Source: CAD feature listing. Evaluate the final solid. Frame: model axes, mm. A direction names the side the tool comes from. Give positions to 0.01 mm unless a question says otherwise; leave off trailing zeros. Write each loop counter-clockwise with the first axis right and the second up, starting at its lowest first coordinate (ties: lowest second). Pieces come first, ordered by that corner, then holes. Notation, with made-up numbers: (50.25, 32.5) -> (61.25, 32.5) arc R18 cw to (61.25, 37.5) -> close; hole circle Ø11 at (37.25, -36). An arc over 180 degrees is marked (long way). Use a Markdown table: item, result. Add a question column.
Autodesk Inventor part; units mm, degrees
ref_plane "Work Plane1" through (0, -12.5, 0) normal (0, -1, 0) x (1, 0, 0)
ref_plane "YZ Plane" through (0, 0, 0) normal (1, 0, 0) x (0, 1, 0)
ref_plane "XZ Plane" through (0, 0, 0) normal (0, 1, 0) x (-1, 0, 0)
sketch "Sketch1" plane through (0, 0, 0) normal (0, 1, 0) x (-1, 0, 0)
  line L0 (0, 0) -> (-150, 0)
  line L1 (-150, 0) -> (-150, -20) construction
  line L2 (-150, -20) -> (0, -37.6327)
  line L3 (0, -37.6327) -> (0, 0) construction
  arc A0 (-150, 0) -> (-150, -20) centre (-150, -10) ccw
  arc A1 (0, -37.6327) -> (0, 0) centre (-6.7783, -18.8163) ccw
  dimension "d0" = 150
  dimension "d1" = 20
  dimension "d3" = 20
extrude "Extrusion1" add sketch "Sketch1" along normal blind 5
sketch "Sketch5" plane through (0, 5, 0) normal (0, 1, 0) x (1, 0, 0)
  line L0 (0, 7) -> (40.3, 7)
  line L1 (40.3, 7) -> (40.3, 27)
  line L2 (40.3, 27) -> (0, 27)
  line L3 (0, 27) -> (0, 7)
  line L4 (0, 0) -> (150, 0)
  arc A0 (0, 37.6327) -> (0, 0) centre (6.7783, 18.8163) ccw
  line L5 (0, 0) -> (0, 37.6327) construction
  dimension "d13" = 40.3
  dimension "d14" = 20
  dimension "d15" = 7
  dimension "d16" = 0
extrude "Extrusion3" cut sketch "Sketch5" against normal blind 5
ref_plane "Work Plane1" through (0, -12.5, 0) normal (0, -1, 0) x (1, 0, 0)
mirror "Mirror1" about plane through (0, -12.5, 0) normal (0, -1, 0) of "Extrusion1"
sketch "Sketch8" plane through (0, 0, 0) normal (0, 0, 1) x (1, 0, 0)
  line L0 (0, 0) -> (40.3, 0)
  line L1 (0, -25) -> (150, -25)
  line L2 (0, 0) -> (40.3767, 0)
  line L3 (40.3767, 0) -> (40.3767, -25)
  line L4 (40.3767, -25) -> (0, -25)
  line L5 (0, -25) -> (0, 0)
extrude "Extrusion4" add sketch "Sketch8" against normal blind 5
sketch "Sketch11" plane through (0, 5, 0) normal (0, 1, 0) x (1, 0, 0)
  circle A0 centre (-3.8458, 11.9975) radius 2
  circle A1 centre (-3.8458, 11.9975) radius 2
  circle A2 centre (-3.8458, 21.9992) radius 2
  circle A3 centre (44.2605, 21.9992) radius 2
  circle A4 centre (-3.8458, 21.9992) radius 2
  circle A5 centre (44.2605, 11.9975) radius 2
  circle A6 centre (44.2605, 21.9992) radius 2
  circle A7 centre (44.2605, 11.9975) radius 2
  point P0 (0, 0)
extrude "Extrusion6" cut sketch "Sketch11" against normal blind 5
sketch "Sketch14" plane through (0, 0, -37.6327) normal (0.1167, 0, -0.9932) x (-0.9932, 0, -0.1167)
  line L0 (-151.0328, -25) -> (0, -25)
  line L1 (-4.3935, 0) -> (-44.3935, 0)
  line L2 (-44.3935, 0) -> (-44.3935, -25)
  line L3 (-44.3935, -25) -> (-4.3935, -25)
  line L4 (-4.3935, -25) -> (-4.3935, 0)
  dimension "d31" = 40
extrude "Extrusion7" add sketch "Sketch14" against normal blind 5
sketch "Sketch17" plane through (0, 5, 0) normal (0, 1, 0) x (1, 0, 0)
  arc A0 (150, 0) -> (150, 20) centre (150, 10) ccw
  line L0 (150, 20) -> (44.0899, 32.4499)
  line L1 (150, 0) -> (150, 20)
  point P0 (0, 0)
extrude "Extrusion10" add sketch "Sketch17" against normal up to surface (35 mm away)
sketch "Sketch18" plane through (0, -30, 0) normal (0, -1, 0) x (1, 0, 0)
  circle A0 centre (10.7396, -16.9983) radius 5
  circle A1 centre (10.7396, -16.9983) radius 2.9
  point P0 (0, 0)
  dimension "d42" = 10
extrude "Extrusion11" add sketch "Sketch18" along normal blind 6 contours A0 | A1
properties part number "Tibia" material "PVC, Unplasticized"
(1) Cut plane A-A on y = -3. Return the cut outline in (x, z), then the cut area to 3 significant figures.
(2) Cut plane B-B on x = 72. Return the cut outline in (y, z).
(3) Material intervals for L1, parallel to Y at x = 127, z = -9; L2, parallel to Y at x = 11, z = -13.5; L3, parallel to Y at x = 9.5, z = -32, sorted ascending.
(4) Mould query, pull axis Z, two halves, no side actions, for faces 1 (the flat face through (20, -12, -5)), 2 (the flat face through (23.921, -12.325, -29.788)), 3 (the flat face through (11, -36, -17)), 4 (the flat face through (24.505, -12.325, -34.753)). Classes: +Z half, -Z half, draft (parallel to the pull), parting line (faces both ways), or undercut.
(5) Cut plane D-D on x = 92. Return the cut outline in (y, z).
(6) Access query for faces 5 (the flat face through (4.076, -12.675, -34.672)), 6 (the flat face through (0, -13, -2)), 7 (the flat face through (40.3, 3, -17)), 8 (the flat face through (67, -25, -14)). Directions: +Z, -Z, +X, -X, +Y, -Y. A direction counts if a zero-diameter tool reaches every point of the face in a straight line with its end or side. Return the directions, or none.
(7) First-contact query: pin 1 Ø10 at (y, z) = (-1, -22) entering from +X; pin 2 Ø4 at (x, y) = (29.5, 3) entering from -Z; pin 3 Ø3.5 at (x, z) = (-3.85, -12) entering from -Y. Flat tips, straight axial feed; report the tip coordinate or a pass-through.
(8) Cut plane C-C on z = -3.5. Return the cut outline in (x, y).
Output:
| question | item | result |
|---|---|---|
| 1 | outline | (0, -5) -> (40.38, -5) -> (40.38, 0) -> (0, 0) -> close; (3.78, -32.15) -> (4.36, -37.12) -> (44.09, -32.45) -> (43.51, -27.49) -> close; (150, -20) arc R10 ccw to (150, 0) -> close |
| 1 | area | 559 mm^2 |
| 2 | outline | (-30, -29.17) -> (-25, -29.17) -> (-25, 0) -> (-30, 0) -> close; (0, -29.17) -> (5, -29.17) -> (5, 0) -> (0, 0) -> close |
| 3 | L1 | -30 to -25, 0 to 5 |
| 3 | L2 | -36 to -25 |
| 3 | L3 | -30 to 5 |
| 4 | face 1 | undercut |
| 4 | face 2 | undercut |
| 4 | face 3 | draft |
| 4 | face 4 | -Z half |
| 5 | outline | (-30, -26.82) -> (-25, -26.82) -> (-25, 0) -> (-30, 0) -> close; (0, -26.82) -> (5, -26.82) -> (5, 0) -> (0, 0) -> close |
| 6 | face 5 | -Z, -X |
| 6 | face 6 | +Z, -Z, -X |
| 6 | face 7 | +Y |
| 6 | face 8 | none |
| 7 | pin 1 | x = 157.14 |
| 7 | pin 2 | z = -34.4 |
| 7 | pin 3 | y = -30 |
| 8 | outline | (-6.08, -30) -> (157.6, -30) -> (157.6, 5) -> (-6.08, 5) -> (-6.08, 0) -> (0, 0) -> (0, -25) -> (-6.08, -25) -> close; hole (40.38, -25) -> (150, -25) -> (150, 0) -> (40.38, 0) -> close |
